Could you check a few things on this model? Use its own coordinates, in mm. Face numbers are marked on the shaded views. A direction names the side the tool comes from. Give positions to 0.01 mm unless a question says otherwise; leave off trailing zeros. Loops run counter-clockwise (first coordinate to the right, second up) from the corner with the lowest first, then second, coordinate; pieces in that order, holes last. Notation, with made-up numbers: (-2, 13.25) -> (20, 13.25) arc R24 cw to (20, 27.25) -> close; hole circle Ø10 at (84.5, 50). An arc over 180 degrees is marked (long way). Write each question's results on one line, items separated by ' | '. Start each with the question number.
Q1. If we section it at C-C, the plane z = 90: List the corners of the cut face in (x, y) for me (3 decimals), plus the area to 3 significant figures.
Q2. We'd pull the mould along X, two halves only. Please class the marked faces 5 and 6: released by +X, released by -X, zero draft, split by the parting line, or undercut.
Q3. Will these pins go through, and if not, where does the flat tip stop? P1, Ø9.5, axis at x = 33.5, y = 10, coming from the +Z side; P2, Ø2.5, axis at x = -7, z = 112, coming from the +Y side; P3, Ø3, axis at x = 48.025, y = 10.5, coming from the +Z side.
Q4. If I drill on line 1 along Z through (x, y) = (48, 5.5); line 2 along Z through (x, y) = (-7, 2.75); line 3 along X through (y, z) = (5, 1.4), over which ranges is the centre line in solid material (lowest first)?
Q5. If we section it at A-A, the plane y = 10.5: Give the number of separate pieces and of enclosed holes in the cut face, plus the area to 3 significant figures.
Q6. Which directions (+Z, -Z, +X, -X, +Y, -Y) give clear straight access to the entire face, cutting with the end or side of a thin tool? Please do the marked faces 1, 2, 3 and 4.
Q7. If we section it at B-B, the plane x = 25: List the corners of the cut face in (y, z) for me.
Autodesk Inventor part; units mm, degrees
ref_plane "Work Plane1" through (0, 0, 80) normal (0, 0, 1) x (1, 0, 0)
ref_plane "YZ Plane" through (0, 0, 0) normal (1, 0, 0) x (0, 1, 0)
ref_plane "XZ Plane" through (0, 0, 0) normal (0, 1, 0) x (-1, 0, 0)
sketch "Sketch1" plane through (0, 0, 0) normal (0, 0, 1) x (1, 0, 0)
  line L0 (0, 0) -> (40, 0)
  line L1 (40, 0) -> (40, 20)
  line L2 (40, 20) -> (0, 20)
  line L3 (0, 20) -> (0, 0)
  dimension "d69" = 20
  dimension "d70" = 40
extrude "Extrusion1" add sketch "Sketch1" along normal blind 5
sketch "Sketch2" plane through (0, 0, 5) normal (0, 0, 1) x (1, 0, 0)
  line L0 (40, 20) -> (0, 20)
  line L1 (0, 0) -> (40, 0)
  line L2 (0, 20) -> (40, 20)
  line L3 (40, 20) -> (40, 0)
  line L4 (40, 0) -> (0, 0)
  line L5 (0, 0) -> (0, 20)
ref_plane "Work Plane1" through (0, 0, 80) normal (0, 0, 1) x (1, 0, 0)
sketch "Sketch3" plane through (0, 0, 80) normal (0, 0, 1) x (1, 0, 0)
  line L0 (10, 15) -> (30, 15)
  line L1 (30, 15) -> (30, 0)
  line L2 (30, 0) -> (10, 0)
  line L3 (10, 0) -> (10, 15)
  line L4 (0, 20) -> (0, 0)
  dimension "d71" = 20
  dimension "d72" = 15
  dimension "d73" = 10
loft "Loft1" add profiles "Sketch3" section 2 edges at (40, 10, 5) (20, 20, 5) (0, 10, 5) (20, 0, 5)
sketch "Sketch4" plane through (0, 0, 80) normal (0, 0, 1) x (1, 0, 0)
  line L0 (53.025, 0) -> (-13.025, 0)
  line L1 (-13.025, 0) -> (-13.025, 15)
  line L2 (-13.025, 15) -> (53.025, 15)
  line L3 (53.025, 15) -> (53.025, 0)
  line L4 (30, 0) -> (10, 0)
  point P0 (0, 0)
  dimension "d16" = 66.05
  dimension "d18" = 15
  dimension "d76" = 0
  dimension "d78" = 13.025
extrude "Extrusion2" add sketch "Sketch4" along normal blind 3
sketch "Sketch5" plane through (0, 0, 83) normal (0, 0, 1) x (1, 0, 0)
  line L0 (-13.025, 0) -> (53.025, 0)
  line L1 (-13.025, 15) -> (-13.025, 0)
  line L2 (53.025, 0) -> (-13.025, 0)
  line L3 (-13.025, 0) -> (-13.025, 3)
  line L4 (-13.025, 3) -> (53.025, 3)
  line L5 (53.025, 3) -> (53.025, 0)
  point P0 (0, 0)
  dimension "d22" = 3
extrude "Extrusion3" add sketch "Sketch5" along normal blind 27
sketch "Sketch6" plane through (0, 0, 110) normal (0, 0, 1) x (1, 0, 0)
  line L0 (53.025, 0) -> (53.025, 15)
  line L1 (-13.025, 15) -> (-13.025, 0)
  line L2 (53.025, 0) -> (-13.025, 0)
  line L3 (-13.025, 0) -> (-13.025, 15)
  line L4 (-13.025, 15) -> (53.025, 15)
  line L5 (53.025, 15) -> (53.025, 0)
  point P0 (0, 0)
extrude "Extrusion4" add sketch "Sketch6" along normal blind 3
sketch "Sketch7" plane through (0, 0, 113) normal (0, 0, 1) x (1, 0, 0)
  circle A0 centre (-8.025, 10.5) radius 1.25
  circle A1 centre (48.025, 10.5) radius 1.25
  line L0 (53.025, 3) -> (-13.025, 3)
  line L1 (-13.025, 3) -> (53.025, 3)
  point P0 (0, 0)
  point P1 (20, 3)
  dimension "d27" = 7.5
  dimension "d28" = 7.5
  dimension "d29" = 56.05
  dimension "d30" = 28.025
  dimension "d31" = 2.5
  dimension "d32" = 2.5
extrude "Extrusion5" cut sketch "Sketch7" against normal blind 35
sketch "Sketch10" plane through (0, 0, 113) normal (0, 0, 1) x (1, 0, 0)
  circle A0 centre (48.025, 10.5) radius 1.25
  circle A1 centre (48.025, 10.5) radius 2.5
  circle A2 centre (-8.025, 10.5) radius 1.25
  circle A3 centre (-8.025, 10.5) radius 2.5
  point P0 (0, 0)
  dimension "d61" = 5
  dimension "d62" = 5
extrude "Extrusion8" cut sketch "Sketch10" against normal blind 1
sketch "Sketch11" plane through (0, 0, 80) normal (0, 0, -1) x (-1, 0, 0)
  circle A0 centre (-48.025, 10.5) radius 1.25
  circle A1 centre (-48.025, 10.5) radius 2.5
  circle A2 centre (8.025, 10.5) radius 1.25
  circle A3 centre (8.025, 10.5) radius 2.5
  point P0 (0, 0)
  dimension "d65" = 5
  dimension "d66" = 5
extrude "Extrusion9" cut sketch "Sketch11" against normal blind 1
sketch "Sketch12" plane through (-13.025, 15, 110) normal (0, 1, 0) x (1, 0, 0)
  line L0 (0, -3) -> (66.05, -3)
  line L1 (10, -3) -> (56.05, -3)
  line L2 (56.05, -3) -> (56.05, 17)
  line L3 (56.05, 17) -> (10, 17)
  line L4 (10, 17) -> (10, -3)
  line L5 (0, 27) -> (0, 0)
  line L6 (66.05, 27) -> (66.05, 0)
  line L7 (66.05, 27) -> (0, 27)
  point P0 (13.025, 110)
  dimension "d79" = 10
  dimension "d80" = 10
  dimension "d81" = 10
extrude "Extrusion10" cut sketch "Sketch12" against normal blind 15
sketch "Sketch15" plane through (0, 0, 0) normal (0, 0, -1) x (-1, 0, 0)
  line L0 (-30, 0) -> (-53.025, 0)
  line L1 (10, 20) -> (-50, 20)
  line L2 (-50, 20) -> (-50, 0)
  line L3 (-50, 0) -> (10, 0)
  line L4 (10, 0) -> (10, 20)
  line L5 (0, 20) -> (0, 0)
  line L6 (-40, 0) -> (-40, 20)
  dimension "d119" = 10
  dimension "d120" = 10
extrude "Extrusion13" add sketch "Sketch15" against normal blind 5 contours L0 L2 L1 L6 | L5 L1 L4 L3
fillet "Fillet1" radius 2 4 edges at (50, 20, 2.5) (50, 0, 2.5) (-10, 20, 2.5) (-10, 0, 2.5)
chamfer "Chamfer1" distance 3 angle 45 2 edges at (10, 7.5, 80) (30, 7.5, 80)
sketch "Sketch17" plane through (0, 20, 5) normal (0, 1, 0) x (1, 0, 0)
  line L0 (40, 0) -> (0, 0)
  line L1 (3.0265, 0) -> (13.0265, -75)
  line L2 (33, -75) -> (7, -75)
  line L3 (36.9735, 0) -> (26.9735, -75)
  line L4 (9.6035, -72.0263) -> (0, 0)
  line L5 (30.3965, -72.0263) -> (40, 0)
  point P0 (0, 5)
  dimension "d138" = 3
  dimension "d139" = 3
extrude "Extrusion15" cut sketch "Sketch17" against normal blind 17
sketch "Sketch16" plane through (0, 0, 0) normal (0, 0, -1) x (-1, 0, 0)
  circle A0 centre (-45, 15) radius 2.2
  circle A1 centre (5, 15) radius 2.2
  circle A2 centre (-20, 5) radius 2.2
  line L0 (-50, 20) -> (-50, 0)
  line L1 (10, 20) -> (-50, 20)
  line L2 (10, 0) -> (10, 20)
  line L3 (-50, 0) -> (10, 0)
  point P0 (0, 0)
  dimension "d123" = 5
  dimension "d124" = 5
  dimension "d125" = 4.4
  dimension "d126" = 4.4
  dimension "d127" = 5
  dimension "d128" = 5
  dimension "d129" = 5
  dimension "d130" = 4.4
  dimension "d134" = 30
extrude "Extrusion16" cut sketch "Sketch16" against normal blind 6 contours A0 | A1 | A2
properties part number "RL_spider_camera_mount"
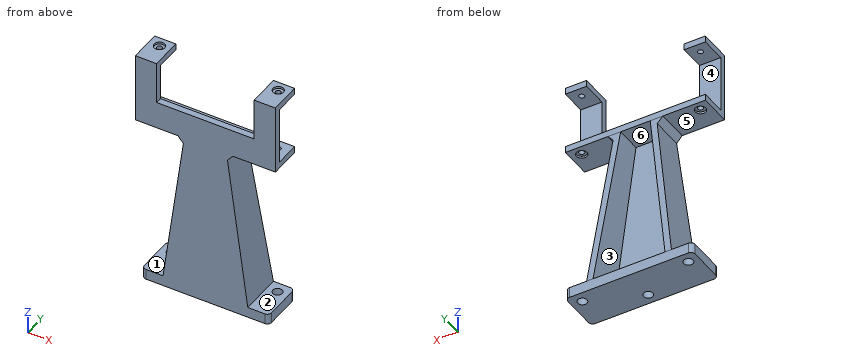
Final values:
1) outline: (-13.025, 0) -> (53.025, 0) -> (53.025, 3) -> (-13.025, 3) -> close | area: 198 mm²
2) face 5: zero draft | face 6: undercut
3) P1: stops at z = 83 | P2: stops at y = 15 | P3: stops at z = 112
4) line 1: z = 0 to 5, 80 to 83, 110 to 113 | line 2: z = 0 to 5, 80 to 113 | line 3: x = -10 to 17.8, 22.2 to 50
5) separate pieces: 7 | enclosed holes: 1 | area: 981 mm²
6) face 1: -X, +Y, -Y | face 2: +X, +Y, -Y | face 3: +Y | face 4: +X, -X, +Y
7) outline: (0, 0) -> (20, 0) -> (20, 5) -> (3, 5) -> (3, 80) -> (15, 80) -> (15, 83) -> (3, 83) -> (3, 93) -> (0, 93) -> close
